Design review of the part built by this model. Coordinates are the model's own, in mm. A direction names the side the tool comes from. Coordinates: 2 decimals unless noted, no trailing zeros. Write each loop counter-clockwise with the first axis right and the second up, starting at its lowest first coordinate (ties: lowest second). Pieces come first, ordered by that corner, then holes. Notation, with made-up numbers: (46, 12) - (77, 12) arc R26 cw to (77, 46) - close; hole circle Ø5 at (-27, 23.5). An arc over 180 degrees is marked (long way). Answer as CSV lines item,"result". Start each with the question number.
Q1. We need section B-B (z = -2.75). Write out the cut boundary in (x, y), plus the area to 3 significant figures.
Q2. Clearance check with a flat-ended pin moving along its axis: pin 1 (2 mm diameter, centred on x = 10, y = 9.5, fed in from -Z). State where the tip first meets the part, or that it passes through.
Q3. Mouldability with a two-part tool opening along Z and no side actions: class faces 6 (the face through (13, 16, -5.93)), 7 (the face through (13, 15, 0)), 8 (the face through (12.52, 6.67, -5.25)), 9 (the face through (0, 7, -9)) as pulls with the +Z half, pulls with the -Z half, needs draft (parallel to the pull), parting line crosses it, or undercut.
Q4. For line 1 along Y through (x, z) = (12, -4.25); line 2 along Z through (x, y) = (19.5, 14.75); line 3 along Z through (x, y) = (21.25, 7.25), list the stretches that pass through material, from the lowest coordinate up. Write a range as [from, to].
Q5. Machinability: for faces 1 (the face through (13, 4, 0)), 2 (the face through (12.52, 18.65, -18.63)), 3 (the face through (13, 7.366, -18)), 4 (the face through (13, 5.893, -16)), 5 (the face through (13, 18, -11.684)), which of the approach directions +Z, -Z, +X, -X, +Y, -Y give a long, thin tool a straight path to every point of the face, cutting with its end or side? Answer none if there is none.
Q6. We need section A-A (y = 3.25). Write out the cut boundary in (x, z), plus the area to 3 significant figures.
Autodesk Inventor part; units mm, degrees
ref_plane "YZ Plane" through (0, 0, 0) normal (1, 0, 0) x (0, 1, 0)
ref_plane "XZ Plane" through (0, 0, 0) normal (0, 1, 0) x (-1, 0, 0)
ref_plane "XY Plane" through (0, 0, 0) normal (0, 0, 1) x (1, 0, 0)
sketch "Sketch2" plane through (0, 0, 0) normal (1, 0, 0) x (0, 1, 0)
  line L0 (1.3843, 0) -> (1.397, 0)
  line L1 (17.653, 0) -> (11.684, 0)
  line L2 (11.684, 0) -> (11.684, -1.397)
  line L3 (11.684, -1.397) -> (13.1572, -1.397)
  line L4 (13.1572, -1.397) -> (13.1572, -4.5085)
  line L5 (13.1572, -4.5085) -> (11.7024, -5.9633)
  line L6 (11.7024, -5.9633) -> (7.3844, -5.9633)
  line L7 (7.3844, -5.9633) -> (5.9296, -4.5085)
  line L8 (5.9296, -4.5085) -> (5.9296, -1.397)
  line L9 (5.9296, -1.397) -> (7.4028, -1.397)
  line L10 (7.4028, -1.397) -> (7.4028, 0)
  line L11 (1.397, 0) -> (7.4028, 0)
  line L12 (11.684, 0) -> (19.05, 0)
  line L13 (5.9633, -7.3476) -> (5.9633, -11.6656)
  line L14 (4.5085, -5.8928) -> (5.9633, -7.3476)
  line L15 (5.9633, -11.6656) -> (4.5085, -13.1204)
  line L16 (1.397, -13.1204) -> (1.397, -11.6472)
  line L17 (4.5085, -13.1204) -> (1.397, -13.1204)
  line L18 (1.397, -11.6472) -> (0, -11.6472)
  line L19 (1.397, -5.8928) -> (4.5085, -5.8928)
  line L20 (0, -7.366) -> (1.397, -7.366)
  line L21 (1.397, -7.366) -> (1.397, -5.8928)
  line L22 (7.3476, -13.0867) -> (11.6656, -13.0867)
  line L23 (5.8928, -14.5415) -> (7.3476, -13.0867)
  line L24 (11.6656, -13.0867) -> (13.1204, -14.5415)
  line L25 (13.1204, -17.653) -> (11.6472, -17.653)
  line L26 (13.1204, -14.5415) -> (13.1204, -17.653)
  line L27 (11.6472, -17.653) -> (11.6472, -19.05)
  line L28 (5.8928, -17.653) -> (5.8928, -14.5415)
  line L29 (7.366, -19.05) -> (7.366, -17.653)
  line L30 (7.366, -17.653) -> (5.8928, -17.653)
  line L31 (13.0867, -11.7024) -> (13.0867, -7.3844)
  line L32 (14.5415, -13.1572) -> (13.0867, -11.7024)
  line L33 (13.0867, -7.3844) -> (14.5415, -5.9296)
  line L34 (17.653, -5.9296) -> (17.653, -7.4028)
  line L35 (14.5415, -5.9296) -> (17.653, -5.9296)
  line L36 (17.653, -7.4028) -> (19.05, -7.4028)
  line L37 (17.653, -13.1572) -> (14.5415, -13.1572)
  line L38 (19.05, -11.684) -> (17.653, -11.684)
  line L39 (17.653, -11.684) -> (17.653, -13.1572)
  line L40 (1.3843, 0) -> (1.397, 0)
  line L41 (19.05, -1.397) -> (19.05, -7.4028)
  line L42 (19.05, -11.684) -> (19.05, -17.653)
  line L43 (17.653, -19.05) -> (11.6472, -19.05)
  line L44 (7.366, -19.05) -> (1.397, -19.05)
  line L45 (0, -17.653) -> (0, -11.6472)
  line L46 (0, -7.366) -> (0, -1.397)
  line L47 (0, -7.366) -> (0, -1.397)
  circle A0 centre (9.525, -9.525) radius 1.5875
  line L48 (1.3843, 0) -> (1.397, 0)
  line L49 (0, -1.397) -> (0, -1.3843)
  arc A1 (1.397, 0) -> (0, -1.397) centre (1.397, -1.397) ccw
  arc A2 (0, -17.653) -> (1.397, -19.05) centre (1.397, -17.653) ccw
  arc A3 (17.653, -19.05) -> (19.05, -17.653) centre (17.653, -17.653) ccw
  arc A4 (19.05, -1.397) -> (17.653, 0) centre (17.653, -1.397) ccw
  point P0 (0, 0)
  dimension "d34" = 7.366
  dimension "d35" = 1.397
  dimension "d37" = 1.4732
  dimension "d38" = 3.1115
  dimension "d39" = 2.0574
  dimension "d40" = 135
  dimension "d41" = 4.318
  dimension "d42" = 2.0574
  dimension "d43" = 1.4732
  dimension "d46" = 1.397
  dimension "d49" = 360
  dimension "d56" = 19.05
  dimension "d58" = 3.175
  dimension "d61" = 1.397
  dimension "d62" = 1.397
  dimension "d63" = 1.397
  dimension "d64" = 1.397
  dimension "d67" = 360
  dimension "d71" = 3.1115
extrude "Extrusion1" add sketch "Sketch2" along normal blind 25.4
properties part number "Extrusion"
Results list:
1,outline,"(0, 0) - (25.4, 0) - (25.4, 5.93) - (0, 5.93) - close; (0, 13.16) - (25.4, 13.16) - (25.4, 19.05) - (0, 19.05) - close"
1,area,"300 mm2"
2,pin 1,"stops at z = -13.09"
3,face 6,"undercut"
3,face 7,"pulls with the +Z half"
3,face 8,"undercut"
3,face 9,"needs draft"
4,line 1,"y = [0, 5.93], [13.16, 19.05]"
4,line 2,"z = [-19.05, -13.16], [-5.93, 0]"
4,line 3,"z = [-19.05, -17.65], [-13.18, -5.83], [-1.4, 0]"
5,face 1,"+Z, +X, -X, +Y, -Y"
5,face 2,"-Z, +X, -X, +Y"
5,face 3,"-Z, +X, -X"
5,face 4,"+X, -X"
5,face 5,"+X, -X, +Y"
6,outline,"(0, -19.05) - (25.4, -19.05) - (25.4, -13.12) - (0, -13.12) - close; (0, -5.89) - (25.4, -5.89) - (25.4, 0) - (0, 0) - close"
6,area,"300 mm2"
